Geometry: final body of the model. Coordinates: model frame, mm. Face numbers are marked on the shaded views. A direction names the side the tool comes from. Round coordinates to 2 decimals unless told otherwise and drop trailing zeros. Loops run counter-clockwise (first coordinate to the right, second up) from the corner with the lowest first, then second, coordinate; pieces in that order, holes last. Notation, with made-up numbers: (58.25, 65.25) -> (108.25, 65.25) arc R12 ccw to (108.25, 83.25) -> close; hole circle Ø9 at (70.25, 60.25). An arc over 180 degrees is marked (long way). Answer in a Markdown table with one row per item.
```python
from build123d import *

# Parameters (mm, degrees)
BOSS_EXTRUDE1_DEPTH = 3
SKETCH5_R           = 1.5875
BOSS_EXTRUDE4_DEPTH = 3.175
BOSS_EXTRUDE5_DEPTH = 10.16
CUT_EXTRUDE1_DEPTH  = 10.16


with BuildPart() as part:
    # Sketch2 → Boss-Extrude1 (new body)
    with BuildSketch(Plane(origin=(0, 0, 0), x_dir=(1, 0, 0), z_dir=(0, 1, 0))):
        with BuildLine():
            Line((0, -3.175), (12.7, -3.175))
            ThreePointArc((12.7, -3.175), (13.915019898, -2.933317516), (14.94506403, -2.24506403))
            Line((14.94506403, -2.24506403), (29.313473824, 12.123345763))
            Line((29.313473824, 12.123345763), (12.123345763, 29.313473824))
            Line((12.123345763, 29.313473824), (-2.24506403, 14.94506403))
            ThreePointArc((-2.24506403, 14.94506403), (-2.933317516, 13.915019898), (-3.175, 12.7))
            Line((-3.175, 12.7), (-3.175, 0))
            ThreePointArc((-3.175, 0), (-2.24506403, -2.24506403), (0, -3.175))
        make_face()
        Polygon((24.029595763, 12.917095763), (12.7, 1.5875), (1.5875, 1.5875), (1.5875, 12.7), (12.917095763, 24.029595763), align=None, mode=Mode.SUBTRACT)
    extrude(amount=BOSS_EXTRUDE1_DEPTH)

    # Sketch5 → Boss-Extrude4 (add)
    with BuildSketch(Plane.XZ):
        with Locations(Location((0, 0, 0), (0, 0, 90))):
            Circle(SKETCH5_R)
        with Locations(Location((12.7, 0, 0), (0, 0, 270))):
            Circle(SKETCH5_R)
        with Locations((0, -12.7)):
            Circle(SKETCH5_R)
    extrude(amount=BOSS_EXTRUDE4_DEPTH)

    # Sketch6 → Boss-Extrude5 (add)
    with BuildSketch(Plane(origin=(0, 3, 0), x_dir=(1, 0, 0), z_dir=(0, 1, 0))):
        with BuildLine():
            Line((12.7, 1.5875), (1.5875, 1.5875))
            Line((1.5875, 1.5875), (1.5875, 12.7))
            Line((1.5875, 12.7), (1.5875, 18.777628061))
            Line((1.5875, 18.777628061), (-2.24506403, 14.94506403))
            ThreePointArc((-2.24506403, 14.94506403), (-2.933317516, 13.915019898), (-3.175, 12.7))
            Line((-3.175, 12.7), (-3.175, 0))
            ThreePointArc((-3.175, 0), (-2.24506403, -2.24506403), (0, -3.175))
            Line((0, -3.175), (12.7, -3.175))
            ThreePointArc((12.7, -3.175), (13.915019898, -2.933317516), (14.94506403, -2.24506403))
            Line((14.94506403, -2.24506403), (18.777628061, 1.5875))
            Line((18.777628061, 1.5875), (12.7, 1.5875))
        make_face()
    extrude(amount=BOSS_EXTRUDE5_DEPTH)

    # Sketch7 → Cut-Extrude1 (cut)
    with BuildSketch(Plane(origin=(0, 13.16, 0), x_dir=(1, 0, 0), z_dir=(0, 1, 0))):
        Polygon((1.5875, 1.5875), (1.5875, 18.777628061), (0, 17.190128061), (0, 0), (17.190128061, 0), (18.777628061, 1.5875), align=None)
    extrude(amount=-CUT_EXTRUDE1_DEPTH, mode=Mode.SUBTRACT)


solid = part.part
```
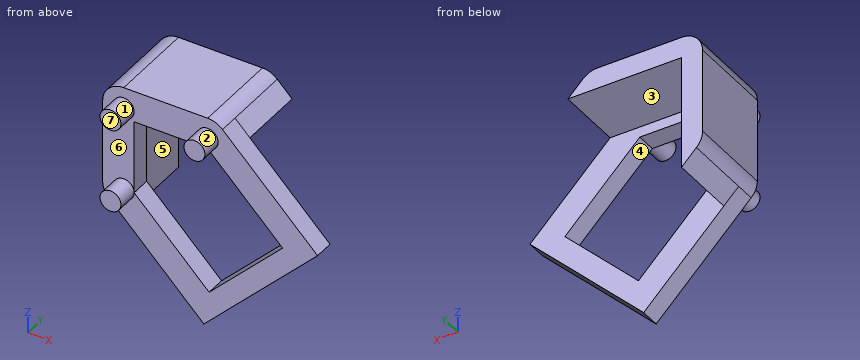
Item 1: Set-up query: the marked faces 4, 5, 6 and 7. Return all of +Z, -Z, +X, -X, +Y, -Y with unobstructed straight access to the full face (end or side cutting, diameter ignored); none if empty.
Ans:
| item | result |
|---|---|
| face 4 | +Y, -Y |
| face 5 | -Z, +X, +Y |
| face 6 | -Y |
| face 7 | +Z, -Z, +X, -X, -Y |
Item 2: Ray query, L1, parallel to X at y = 5, z = -3 (3 decimals); L2, parallel to Y at x = 14, z = -25.5; L3, parallel to Z at x = 18.5, y = 0.5. Return the intervals inside material, ascending.
Ans:
| item | result |
|---|---|
| L1 | -3.175 to 0 |
| L2 | 0 to 3 |
| L3 | -22.94 to -18.45, -7.39 to -1.31 |
Item 3: Section query C-C, the plane x = 4.5. Output: boundary loops of the cut face in (y, z) (1 decimal).
Ans:
| item | result |
|---|---|
| outline | (0, -21.7) -> (3, -21.7) -> (3, -15.6) -> (0, -15.6) -> close; (0, -1.6) -> (3, -1.6) -> (3, 0) -> (13.2, 0) -> (13.2, 3.2) -> (0, 3.2) -> close |
Item 4: Section query B-B, the plane z = -3. Output: boundary loops of the cut face in (x, y) (1 decimal), and give its area (3 significant figures).
Ans:
| item | result |
|---|---|
| outline | (-3.2, 0) -> (1.6, 0) -> (1.6, 3) -> (0, 3) -> (0, 13.2) -> (-3.2, 13.2) -> close; (14.1, 0) -> (20.2, 0) -> (20.2, 3) -> (14.1, 3) -> close |
| area | 64.8 mm2 |
Item 5: Mould query, pull axis Z, two halves, no side actions, for the marked faces 1, 2 and 3. Classes: released by +Z, released by -Z, zero draft, split by the parting line, or undercut.
Ans:
| item | result |
|---|---|
| face 1 | undercut |
| face 2 | split by the parting line |
| face 3 | released by -Z |
Item 6: First-contact query: P1, Ø1.5, axis at y = 1, z = -5.5, coming from the +X side; P2, Ø3, axis at y = 7.5, z = -9.5, coming from the +X side; P3, Ø1.5, axis at x = 9.5, y = 1.5, coming from the -Z side. Flat tips, straight axial feed; report the tip coordinate or a pass-through.
Ans:
| item | result |
|---|---|
| P1 | x = 23.44 |
| P2 | x = 0 |
| P3 | z = -27.44 |
Item 7: Section query D-D, the plane y = 10.25. Output: boundary loops of the cut face in (x, z) (3 decimals).
Ans:
| item | result |
|---|---|
| outline | (-3.175, -12.7) arc R3.175 ccw to (-2.245, -14.945) -> (0, -17.19) -> (0, 0) -> (17.19, 0) -> (14.945, 2.245) arc R3.175 ccw to (12.7, 3.175) -> (0, 3.175) arc R3.175 ccw to (-3.175, 0) -> close |
